from build123d import *

# Parameters (mm, degrees)
SKETCH1_R           = 3.2639
BOSS_EXTRUDE1_DEPTH = 4.7752


with BuildPart() as part:
    # Sketch1 → Boss-Extrude1 (new body)
    with BuildSketch(Plane.XY):
        with BuildLine():
            Line((-38.1, 0), (38.1, 0))
            Line((38.1, 0), (38.1, 24.638))
            Line((38.1, 24.638), (14.7066, 24.638))
            ThreePointArc((14.7066, 24.638), (13.018311849, 25.337311849), (12.319, 27.0256))
            Line((12.319, 27.0256), (12.319, 76.2))
            Line((12.319, 76.2), (-12.319, 76.2))
            Line((-12.319, 76.2), (-12.319, 27.0256))
            ThreePointArc((-12.319, 27.0256), (-13.018311849, 25.337311849), (-14.7066, 24.638))
            Line((-14.7066, 24.638), (-38.1, 24.638))
            Line((-38.1, 24.638), (-38.1, 0))
        make_face()
        with Locations((25.4, 12.7)):
            Circle(SKETCH1_R, mode=Mode.SUBTRACT)
        with Locations((0, 38.1)):
            Circle(SKETCH1_R, mode=Mode.SUBTRACT)
        with Locations((0, 63.5)):
            Circle(SKETCH1_R, mode=Mode.SUBTRACT)
        with Locations((0, 12.7)):
            Circle(SKETCH1_R, mode=Mode.SUBTRACT)
        with Locations((-25.4, 12.7)):
            Circle(SKETCH1_R, mode=Mode.SUBTRACT)
    extrude(amount=BOSS_EXTRUDE1_DEPTH)


solid = part.part
Part model, mm, in its own coordinate system. A direction names the side the tool comes from. Round coordinates to 2 decimals unless told otherwise and drop trailing zeros. Write each loop counter-clockwise with the first axis right and the second up, starting at its lowest first coordinate (ties: lowest second). Pieces come first, ordered by that corner, then holes. Notation, with made-up numbers: M 33.5,24.25 L 82.5,24.25 A21 ccw 82.5,52.25 Z; hole C 80,66 d3. An arc over 180 degrees is marked long. Return JSON: item names as keys, results as strings. Group by question number.
(1) Which spindle directions (+Z, -Z, +X, -X, +Y, -Y) get a long thin tool onto all of the face, cutting with end or side? Do faces 4 (the face through (27, 24.638, 2)), 5 (the face through (28.415, 11.45, 2.354)), 6 (the face through (-12.319, 52, 2)). Say none if no direction does.
(2) Two-plate mould, pull along Y, no slides. Class faces 1 (the face through (1.755, 66.252, 2.354)), 2 (the face through (38.1, 12, 2)), 3 (the face through (-13, 25.356, 2.354)): +Y half, -Y half, draft (parallel to the pull), parting line (faces both ways), or undercut.
(3) Pin check, flat tips, straight feed: pin 1 Ø1.4 at (x, z) = (27.5, 1.5) entering from +Y; pin 2 Ø1.4 at (y, z) = (42, 3) entering from +X. Stop position of each tip, or through.
(4) Drill centre lines: probe 1 along Y at (x, z) = (0, 2.4); probe 2 along Y at (x, z) = (-0.5, 4.2); probe 3 along Y at (x, z) = (25.4, 2.4). Where is each one in solid material? Low to high.
(5) Saw through at D-D on x = 0. Write the cut outline in (y, z), then the cut area to 3 significant figures.
(6) Saw through at A-A on x = 25.4. Write the cut outline in (y, z), then the cut area to 3 significant figures.
(7) Saw through at C-C on z = 3.55. Write the cut outline in (x, y), then the cut area to 3 significant figures.
(8) Saw through at B-B on y = 63.5. Write the cut outline in (x, z), then the cut area to 3 significant figures.
Returned:
{
 "1": {"face 4": "+Z, -Z, +X, +Y", "face 5": "+Z, -Z", "face 6": "+Z, -Z, -X, +Y"},
 "2": {"face 1": "undercut", "face 2": "draft", "face 3": "+Y half"},
 "3": {"pin 1": "y = 24.64", "pin 2": "x = 12.32"},
 "4": {"probe 1": "0 to 9.44, 15.96 to 34.84, 41.36 to 60.24, 66.76 to 76.2", "probe 2": "0 to 9.47, 15.93 to 34.87, 41.33 to 60.27, 66.73 to 76.2", "probe 3": "0 to 9.44, 15.96 to 24.64"},
 "5": {"outline": "M 0,0 L 9.44,0 L 9.44,4.78 L 0,4.78 Z; M 15.96,0 L 34.84,0 L 34.84,4.78 L 15.96,4.78 Z; M 41.36,0 L 60.24,0 L 60.24,4.78 L 41.36,4.78 Z; M 66.76,0 L 76.2,0 L 76.2,4.78 L 66.76,4.78 Z", "area": "270 mm²"},
 "6": {"outline": "M 0,0 L 9.44,0 L 9.44,4.78 L 0,4.78 Z; M 15.96,0 L 24.64,0 L 24.64,4.78 L 15.96,4.78 Z", "area": "86.5 mm²"},
 "7": {"outline": "M -38.1,0 L 38.1,0 L 38.1,24.64 L 14.71,24.64 A2.39 cw 12.32,27.03 L 12.32,76.2 L -12.32,76.2 L -12.32,27.03 A2.39 cw -14.71,24.64 L -38.1,24.64 Z; hole C -25.4,12.7 d6.53; hole C 0,12.7 d6.53; hole C 0,38.1 d6.53; hole C 0,63.5 d6.53; hole C 25.4,12.7 d6.53", "area": "2,980 mm²"},
 "8": {"outline": "M -12.32,0 L -3.26,0 L -3.26,4.78 L -12.32,4.78 Z; M 3.26,0 L 12.32,0 L 12.32,4.78 L 3.26,4.78 Z", "area": "86.5 mm²"}
}
